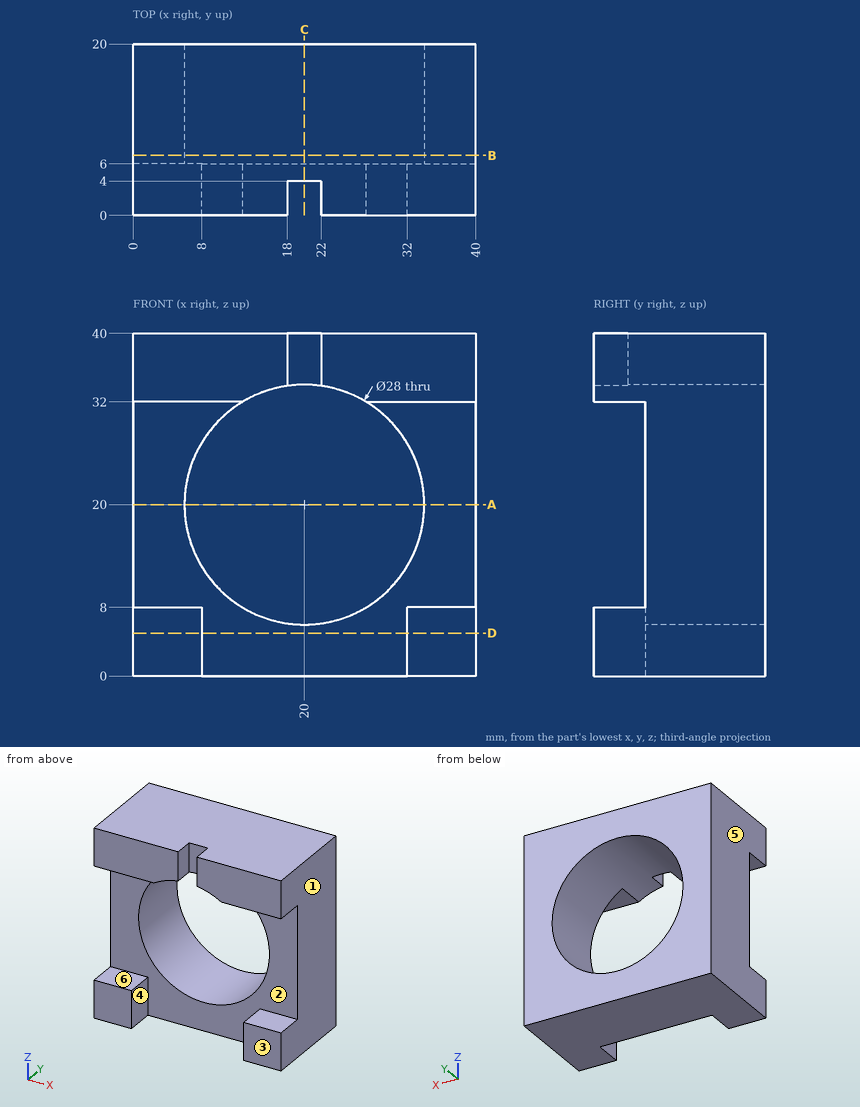
Here's the drawing with two shaded views (mm, measured from the low corner). I have some questions. A direction names the side the tool comes from. Coordinates: 2 decimals unless noted, no trailing zeros. Order: outer loops, then holes, each group sorted by start corner. A loop starts at its lowest first (then second) coordinate and runs counter-clockwise, first axis right, second up. Notation, with made-up numbers: M 55,48 L 64,48 A21 cw 64,87 Z; hole C 7.25,43.25 d8. An arc over 180 degrees is marked long. Answer as CSV lines item,"result".
Item 1: On a 3-axis mill with a long thin cutter (end or side, diameter ignored), from which of +Z, -Z, +X, -X, +Y, -Y can I reach the whole of each face in a straight line? I mean the marked faces 5 and 6. Say none if no direction works.
Results found:
face 5,"+Z, -Z, -X, +Y, -Y"
face 6,"+X, -X, -Y"
Item 2: Imagine slicing it at C-C on x = 20. Write out the boundary of the cut face in (y, z), plus the area to 3 significant figures.
Results found:
outline,"M 4,34 L 20,34 L 20,40 L 4,40 Z; M 6,0 L 20,0 L 20,6 L 6,6 Z"
area,"180 mm2"
Item 3: For pin 1 (2 mm diameter, centred on x = 20.5, z = 37.5, fed in from -Y), with a flat end and sliding along its axis, tell me the tip position at first contact or that it passes through.
Results found:
pin 1,"y = 4"
Item 4: If I drill on line 1 (X direction, y = 9.75, z = 8); line 2 (X direction, y = 14.5, z = 20), over which ranges is the centre line in solid material (lowest first)?
Results found:
line 1,"0 to 12.79, 27.21 to 40"
line 2,"0 to 6, 34 to 40"
Item 5: Imagine slicing it at A-A on z = 20. Write out the boundary of the cut face in (x, y), plus the area to 3 significant figures.
Results found:
outline,"M 0,6 L 6,6 L 6,20 L 0,20 Z; M 34,6 L 40,6 L 40,20 L 34,20 Z"
area,"168 mm2"
Item 6: We'd pull the mould along X, two halves only. Please class the marked faces 1, 2, 3 and 4: +X half, -X half, draft (parallel to the pull), parting line (faces both ways), or undercut.
Results found:
face 1,"+X half"
face 2,"undercut"
face 3,"draft"
face 4,"undercut"
Item 7: Imagine slicing it at B-B on y = 7. Write out the boundary of the cut face in (x, z).
Results found:
outline,"M 0,0 L 40,0 L 40,40 L 0,40 Z; hole C 20,20 d28"
Item 8: Imagine slicing it at D-D on z = 5. Write out the boundary of the cut face in (x, y), plus the area to 3 significant figures.
Results found:
outline,"M 0,0 L 8,0 L 8,6 L 32,6 L 32,0 L 40,0 L 40,20 L 0,20 Z"
area,"656 mm2"
